```python
from build123d import *

# Parameters (mm, degrees)
SKETCH3_R               = 1.5
SKETCH3_R_2             = 1
BOSS_EXTRUDE2_DEPTH     = 3
SCALE1_SCALE            = 2
CUT_EXTRUDE1_DEPTH      = 236.835290083
CUT_EXTRUDE1_DEPTH_BACK = 236.835290083


with BuildPart() as part:
    # Sketch3 → Boss-Extrude2 (new body)
    with BuildSketch(Plane.YZ):
        with BuildLine():
            ThreePointArc((118.150026657, 100.656257205), (107.173519636, 113.210773098), (93.56234312, 122.845888539))
            ThreePointArc((93.56234312, 122.845888539), (81.890744338, 136.842623997), (100.108836706, 136.356895566))
            ThreePointArc((100.108836706, 136.356895566), (117.223173705, 124.346501771), (130.920746245, 108.550090897))
            ThreePointArc((130.920746245, 108.550090897), (133.266943269, 90.477177984), (118.150026657, 100.656257205))
        make_face()
        with Locations(Location((128.009104434, 98.9833599, 0), (0, 0, 270))):
            Circle(SKETCH3_R, mode=Mode.SUBTRACT)
        with Locations(Location((90.890008855, 132.482206797, 0), (0, 0, 270))):
            Circle(SKETCH3_R_2, mode=Mode.SUBTRACT)
    extrude(amount=BOSS_EXTRUDE2_DEPTH)


with BuildPart() as part_1:
    # Scale1: scaled about (1.5, 110.52343824, 117.054422993)
    add(part.part.scale(SCALE1_SCALE).moved(Location((-1.5, -110.52343824, -117.054422993))))

    # Sketch4 → Cut-Extrude1 (cut, two sides: drawn at the far end of the back side and taken through both)
    # profile 1 of 2: a face of its own
    with BuildSketch(Plane(origin=(-1.5, 0, 0), x_dir=(0, -1, 0), z_dir=(-1, 0, 0)).offset(-CUT_EXTRUDE1_DEPTH_BACK)):
        with BuildLine():
            ThreePointArc((-97.213316268, 162.951526918), (-130.622678549, 139.062399665), (-157.803069224, 108.271130585))
            ThreePointArc((-157.803069224, 108.271130585), (-161.544389081, 55.566493456), (-115.500216043, 81.48386945))
            ThreePointArc((-115.500216043, 81.48386945), (-97.123831652, 101.943304086), (-74.892452954, 118.131131925))
            ThreePointArc((-74.892452954, 118.131131925), (-44.402388035, 161.28356164), (-97.213316268, 162.951526918))
        make_face()
        with BuildLine():
            ThreePointArc((-125.776615074, 84.258091416), (-103.823601031, 109.367123202), (-76.601248, 128.637354084))
            ThreePointArc((-76.601248, 128.637354084), (-53.258050437, 156.630825002), (-89.694235172, 155.659368138))
            ThreePointArc((-89.694235172, 155.659368138), (-123.922909169, 131.638580549), (-151.318054249, 100.045758801))
            ThreePointArc((-151.318054249, 100.045758801), (-156.010448298, 63.899932976), (-125.776615074, 84.258091416))
        make_face(mode=Mode.SUBTRACT)
    # profile 2 of 2: a face of its own
    with BuildSketch(Plane(origin=(-1.5, 0, 0), x_dir=(0, -1, 0), z_dir=(-1, 0, 0)).offset(-CUT_EXTRUDE1_DEPTH_BACK)):
        with BuildLine():
            ThreePointArc((-151.318054249, 100.045758801), (-156.010448298, 63.899932976), (-125.776615074, 84.258091416))
            ThreePointArc((-125.776615074, 84.258091416), (-103.823601031, 109.367123202), (-76.601248, 128.637354084))
            ThreePointArc((-76.601248, 128.637354084), (-53.258050437, 156.630825002), (-89.694235172, 155.659368138))
            ThreePointArc((-89.694235172, 155.659368138), (-123.922909169, 131.638580549), (-151.318054249, 100.045758801))
        make_face()
        with BuildLine():
            ThreePointArc((-150.898316566, 83.520302039), (-148.562598659, 75.755899696), (-140.624556205, 77.407869396))
            ThreePointArc((-140.624556205, 77.407869396), (-107.93501235, 113.922858215), (-68.268560869, 142.706939107))
            ThreePointArc((-68.268560869, 142.706939107), (-65.87894024, 150.571004751), (-73.580432021, 153.441691001))
            add(Edge.make_bspline(
                [(-150.898316566, 83.520302039), (-145.205189888, 95.315934641), (-127.744788656, 114.843857064), (-100.777949871, 137.161096472), (-82.38983998, 149.740882267), (-73.580432021, 153.441691001)],
                knots=[0, 0, 0, 0, 0.370027271, 0.730223157, 1, 1, 1, 1], degree=3))
        make_face(mode=Mode.SUBTRACT)
    extrude(amount=CUT_EXTRUDE1_DEPTH + CUT_EXTRUDE1_DEPTH_BACK, mode=Mode.SUBTRACT)


solid = part_1.part
```
CAD build for the part. Positions are in the model's coordinates, mm. Round coordinates to 2 decimals unless told otherwise and drop trailing zeros. Return JSON: item names as keys, results as strings. Group by question number.
Item 1: Flat gauge pins, fed straight in: pin 1 Ø1 at (x, y) = (3.5, 142) entering from +Z; pin 2 Ø1.5 at (x, z) = (3, 143.5) entering from +Y; pin 3 Ø1 at (x, z) = (-1, 91.5) entering from -Y. Where does each tip first touch, or does it go through?
Item 2: Mould opens along Z. For faces 1 (the face through (1.458, 148.024, 79.3)), 2 (the face through (1.542, 65.824, 150.457)), 3 (the face through (-1.5, 112, 115)) say: +Z half, -Z half, draft (parallel to the pull), parting line (faces both ways), or undercut.
Item 3: Probe probe 1 along Y at (x, z) = (3, 79); probe 2 along Y at (x, z) = (2, 148.5); probe 3 along Z at (x, y) = (-1, 143.5). List the from-to ranges inside material, lowest first.
Item 4: Band-saw the part on A-A on x = 2. State how many separate pieces and enclosed holes the cut face has, plus the area to 3 significant figures.
Resolved:
{
 "1": {"pin 1": "stops at z = 98.43", "pin 2": "stops at y = 92.28", "pin 3": "stops at y = 129.21"},
 "2": {"face 1": "undercut", "face 2": "parting line", "face 3": "draft"},
 "3": {"probe 1": "y = 139.47 to 143.18, 147.81 to 151.18", "probe 2": "y = 65.29 to 69.35, 73.17 to 83.38", "probe 3": "z = 75.25 to 78.67, 83.15 to 95.77"},
 "4": {"separate pieces": "1", "enclosed holes": "2", "area": "1,390 mm²"}
}
